```python
from build123d import *

# Parameters (mm, degrees)
SKETCH2_W               = 30
SKETCH2_H               = 30
BOSS_EXTRUDE1_DEPTH     = 60
FILLET1_R               = 10
SKETCH3_W               = 40
SKETCH3_H               = 25
CUT_EXTRUDE1_DEPTH      = 69.738635424
SKETCH6_W               = 30
SKETCH6_H               = 40
BOSS_EXTRUDE2_DEPTH     = 125
SKETCH7_W               = 30
SKETCH7_H               = 10
BOSS_EXTRUDE3_DEPTH     = 10
FILLET2_START           = -16
FILLET2_DEPTH           = 32
FILLET2_START_2         = -15
FILLET2_2_DEPTH         = 30
SKETCH8_W               = 25
SKETCH8_H               = 70
CUT_EXTRUDE2_DEPTH      = 156.241746963
SKETCH12_W              = 30
SKETCH12_H              = 7.5
BOSS_EXTRUDE4_DEPTH     = 65
CUT_EXTRUDE3_DEPTH      = 212.541958013
CUT_EXTRUDE3_DEPTH_BACK = 7.5
SKETCH13_R              = 2.5
SKETCH13_W              = 20
SKETCH13_H              = 42
SKETCH14_W              = 20
SKETCH14_H              = 54
CUT_EXTRUDE4_DEPTH      = 6
SKETCH15_R              = 5
BOSS_EXTRUDE5_DEPTH     = 10
CUT_EXTRUDE5_REACH      = 213.542


with BuildPart() as part:
    # Sketch2 → Boss-Extrude1 (new body)
    with BuildSketch(Plane.XY):
        Rectangle(SKETCH2_W, SKETCH2_H)
        with BuildLine():
            ThreePointArc((5.25, 0), (-2.561737691, -4.582575695), (-2.75, 4.472135955))
            Line((-2.75, 4.472135955), (-2.75, 8.5))
            Line((-2.75, 8.5), (0, 8.5))
            Line((0, 8.5), (2.75, 8.5))
            Line((2.75, 8.5), (2.75, 4.472135955))
            ThreePointArc((2.75, 4.472135955), (4.582575695, 2.561737691), (5.25, 0))
        make_face(mode=Mode.SUBTRACT)
    extrude(amount=BOSS_EXTRUDE1_DEPTH)

    # Fillet1
    fillet1_edges = [part.edges().sort_by_distance(p)[0] for p in [
        (15, -15, 30),
        (-15, -15, 30),
    ]]
    fillet(fillet1_edges, radius=FILLET1_R)

    # Sketch3 → Cut-Extrude1 (cut, through all)
    with BuildSketch(Plane.ZY.offset(15)):
        with Locations((30, -2.5)):
            Rectangle(SKETCH3_W, SKETCH3_H)
    extrude(amount=-CUT_EXTRUDE1_DEPTH, mode=Mode.SUBTRACT)

    # Sketch6 → Boss-Extrude2 (add)
    with BuildSketch(Plane(origin=(0, 15, 0), x_dir=(1, 0, 0), z_dir=(0, 1, 0))):
        with Locations((0, -30)):
            Rectangle(SKETCH6_W, SKETCH6_H)
    extrude(amount=BOSS_EXTRUDE2_DEPTH)

    # Sketch7 → Boss-Extrude3 (add)
    with BuildSketch(Plane(origin=(0, 15, 0), x_dir=(1, 0, 0), z_dir=(0, 1, 0))):
        with Locations((0, -5)):
            Rectangle(SKETCH7_W, SKETCH7_H)
        with Locations((0, -55)):
            Rectangle(SKETCH7_W, SKETCH7_H)
    extrude(amount=BOSS_EXTRUDE3_DEPTH)

    # Fillet2: read off the stored shape, not the designer's step
    # Fillet2 outline → Fillet2 (cut)
    with BuildSketch(Plane.YZ.offset(FILLET2_START)):
        with BuildLine():
            ThreePointArc((25, 5), (23.535533906, 1.464466094), (20, 0))
            Line((20, 0), (25, 0))
            Line((25, 0), (25, 5))
        make_face()
        with BuildLine():
            Line((25, 60), (20, 60))
            ThreePointArc((20, 60), (23.535533906, 58.535533906), (25, 55))
            Line((25, 55), (25, 60))
        make_face()
    extrude(amount=FILLET2_DEPTH, mode=Mode.SUBTRACT)

    # Fillet2 2 outline → Fillet2 2 (add)
    with BuildSketch(Plane.YZ.offset(FILLET2_START_2)):
        with BuildLine():
            Line((25, 10), (25, 5))
            ThreePointArc((25, 5), (26.464466094, 8.535533906), (30, 10))
            Line((30, 10), (25, 10))
        make_face()
        with BuildLine():
            ThreePointArc((30, 50), (26.464466094, 51.464466094), (25, 55))
            Line((25, 55), (25, 50))
            Line((25, 50), (30, 50))
        make_face()
    extrude(amount=FILLET2_2_DEPTH)

    # Sketch8 → Cut-Extrude2 (cut, through all)
    with BuildSketch(Plane(origin=(15, 0, 0), x_dir=(0, 0, -1), z_dir=(1, 0, 0))):
        with Locations((-30, 105)):
            Rectangle(SKETCH8_W, SKETCH8_H)
    extrude(amount=-CUT_EXTRUDE2_DEPTH, mode=Mode.SUBTRACT)

    # Sketch12 → Boss-Extrude4 (add)
    with BuildSketch(Plane(origin=(0, 140, 0), x_dir=(1, 0, 0), z_dir=(0, 1, 0))):
        with Locations((0, -13.75)):
            Rectangle(SKETCH12_W, SKETCH12_H)
        with Locations((0, -46.25)):
            Rectangle(SKETCH12_W, SKETCH12_H)
    extrude(amount=BOSS_EXTRUDE4_DEPTH)

    # Sketch13 → Cut-Extrude3 (cut, two sides: drawn at the far end of the back side and taken through both)
    with BuildSketch(Plane.XY.offset(50).offset(-CUT_EXTRUDE3_DEPTH_BACK)):
        with Locations((-5.125, 192)):
            Circle(SKETCH13_R)
        with Locations((5.125, 192)):
            Circle(SKETCH13_R)
        with Locations((-5.125, 144)):
            Circle(SKETCH13_R)
        with Locations((5.125, 144)):
            Circle(SKETCH13_R)
        with Locations((0, 168)):
            Rectangle(SKETCH13_W, SKETCH13_H)
    extrude(amount=CUT_EXTRUDE3_DEPTH + CUT_EXTRUDE3_DEPTH_BACK, mode=Mode.SUBTRACT)

    # Sketch14 → Cut-Extrude4 (cut)
    with BuildSketch(Plane.XY.offset(50)):
        with Locations((0, 168)):
            Rectangle(SKETCH14_W, SKETCH14_H)
    extrude(amount=-CUT_EXTRUDE4_DEPTH, mode=Mode.SUBTRACT)

    # Sketch15 → Boss-Extrude5 (add)
    with BuildSketch(Plane(origin=(0, 0, 10), x_dir=(-1, 0, 0), z_dir=(0, 0, -1))):
        with Locations(Location((0, 179, 0), (0, 0, 180))):
            Circle(SKETCH15_R)
    extrude(amount=BOSS_EXTRUDE5_DEPTH)

    # Cut-Extrude5: up to this face of the body (flat: up to its plane)
    cut_extrude5_end = Plane(part.part.faces().sort_by_distance((0, 104.420863309, 50))[0])
    # Sketch18 → Cut-Extrude5 (cut, up to the picked face)
    with BuildSketch(Plane(origin=(0, 0, 10), x_dir=(-1, 0, 0), z_dir=(0, 0, -1)), mode=Mode.PRIVATE) as cut_extrude5_sk1:
        with BuildLine():
            Line((-15, 195.093476939), (-15, 205))
            Line((-15, 205), (15, 205))
            Line((15, 205), (15, 195.093476939))
            ThreePointArc((15, 195.093476939), (0, 201), (-15, 195.093476939))
        make_face()
    cut_extrude5_tool1 = split(extrude(cut_extrude5_sk1.sketch, amount=-CUT_EXTRUDE5_REACH, mode=Mode.PRIVATE), bisect_by=cut_extrude5_end, keep=Keep.BOTH, mode=Mode.PRIVATE)
    add(cut_extrude5_tool1.solids().sort_by(Axis((0, 201.823225, 10), (0, 0, 1)))[0], mode=Mode.SUBTRACT)


solid = part.part
```
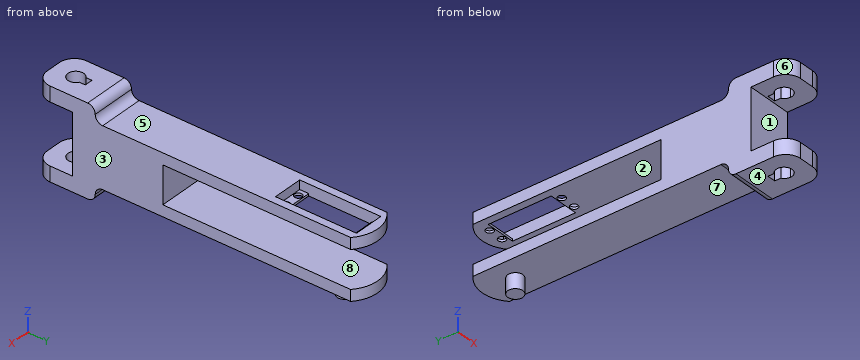
Here's how the part is built. I have some questions about the finished solid (model axes, mm). Face numbers are marked on the shaded views. A direction names the side the tool comes from. Round coordinates to 2 decimals unless told otherwise and drop trailing zeros. Loops run counter-clockwise (first coordinate to the right, second up) from the corner with the lowest first, then second, coordinate; pieces in that order, holes last. Notation, with made-up numbers: (-23.5, 64.25) -> (-19.5, 64.25) arc R29 cw to (-19.5, 91.25) -> close; hole circle Ø8 at (-5.5, 28.5). An arc over 180 degrees is marked (long way). Answer as CSV lines item,"result". Start each with the question number.
1. I need wall thicknesses on probe 1 along X at (y, z) = (0, 55.5); probe 2 along Z at (x, y) = (-11, 98.5); probe 3 along X at (y, z) = (192, 43.4) (3 decimals). Which ranges of each line are inside material? Lowest first, please. Write a range as from..to.
2. Imagine slicing it at D-D on x = 0. State how many separate pieces and enclosed holes the cut face has, plus the area to 3 significant figures.
3. If we mould it in two halves opening along Z, with no side actions, what happens to the marked faces 6, 7 and 8? For each: pulls with the +Z half, pulls with the -Z half, needs draft (parallel to the pull), parting line crosses it, or undercut.
4. For the marked faces 1, 2, 3, 4 and 5, which set-ups out of +Z, -Z, +X, -X, +Y, -Y let a thin tool reach every point of the face, with its end or its side?
5. Imagine slicing it at C-C on z = 52.5. Write out the boundary of the cut face in (x, y), plus the area to 3 significant figures.
6. Imagine slicing it at B-B on y = 108.5. Write out the boundary of the cut face in (x, z).
7. Imagine slicing it at A-A on y = 144. Write out the boundary of the cut face in (x, z) (3 decimals).
8. I'm going to push flat-ended pins straight in: P1, Ø4, axis at x = 11, y = 95.5, coming from the +Z side; P2, Ø15, axis at x = 4, y = 130.5, coming from the -Z side; P3, Ø8, axis at x = 1.5, z = 32, coming from the +Y side. Where does each tip first touch, or does it pass through?
Solution:
1,probe 1,"-15..-5.25, 5.25..15"
1,probe 2,"10..17.5, 42.5..50"
1,probe 3,"-15..-7.625, -2.625..2.625, 7.625..15"
2,separate pieces,"4"
2,enclosed holes,"0"
2,area,"4,600 mm²"
3,face 6,"needs draft"
3,face 7,"pulls with the -Z half"
3,face 8,"undercut"
4,face 1,"+X, -X, -Y"
4,face 2,"+X, -X, +Y"
4,face 3,"+Z, -Z, +X, +Y, -Y"
4,face 4,"-Z, +X, -X, +Y, -Y"
4,face 5,"+Z, +X, -X, +Y"
5,outline,"(-15, -5) arc R10 ccw to (-5, -15) -> (5, -15) arc R10 ccw to (15, -5) -> (15, 25.67) -> (-15, 25.67) -> close; hole (-2.75, 4.47) arc R5.25 ccw (long way) to (2.75, 4.47) -> (2.75, 8.5) -> (-2.75, 8.5) -> close"
5,area,"1,070 mm²"
6,outline,"(-15, 10) -> (15, 10) -> (15, 17.5) -> (-15, 17.5) -> close; (-15, 42.5) -> (15, 42.5) -> (15, 50) -> (-15, 50) -> close"
7,outline,"(-15, 10) -> (15, 10) -> (15, 17.5) -> (-15, 17.5) -> close; (-15, 42.5) -> (-7.625, 42.5) -> (-7.625, 44) -> (-10, 44) -> (-10, 50) -> (-15, 50) -> close; (-2.625, 42.5) -> (2.625, 42.5) -> (2.625, 44) -> (-2.625, 44) -> close; (7.625, 42.5) -> (15, 42.5) -> (15, 50) -> (10, 50) -> (10, 44) -> (7.625, 44) -> close"
8,P1,"z = 50"
8,P2,"z = 10"
8,P3,"y = 70"
